from build123d import *

# Parameters (mm, degrees)
SKETCH1_W           = 8
SKETCH1_H           = 8
BOSS_EXTRUDE1_DEPTH = 2
SKETCH2_W           = 6
SKETCH2_H           = 6
BOSS_EXTRUDE2_DEPTH = 5
FILLET1_R           = 1
SKETCH3_W           = 4
SKETCH3_H           = 4
BOSS_EXTRUDE3_DEPTH = 2.2
FILLET2_R           = 0.5


with BuildPart() as part:
    # Sketch1 → Boss-Extrude1 (new body)
    with BuildSketch(Plane(origin=(0, 0, 0), x_dir=(1, 0, 0), z_dir=(0, 1, 0))):
        Rectangle(SKETCH1_W, SKETCH1_H)
    extrude(amount=BOSS_EXTRUDE1_DEPTH)

    # Sketch2 → Boss-Extrude2 (add)
    with BuildSketch(Plane(origin=(0, 2, 0), x_dir=(1, 0, 0), z_dir=(0, 1, 0))):
        Rectangle(SKETCH2_W, SKETCH2_H)
    extrude(amount=BOSS_EXTRUDE2_DEPTH)

    # Fillet1
    fillet1_edges = [part.edges().sort_by_distance(p)[0] for p in [
        (3, 4.5, 3),
        (3, 4.5, -3),
        (-3, 4.5, -3),
        (-3, 4.5, 3),
    ]]
    fillet(fillet1_edges, radius=FILLET1_R)

    # Sketch3 → Boss-Extrude3 (add)
    with BuildSketch(Plane(origin=(0, 0, 0), x_dir=(-1, 0, 0), z_dir=(0, -1, 0))):
        Rectangle(SKETCH3_W, SKETCH3_H)
    extrude(amount=BOSS_EXTRUDE3_DEPTH)

    # Fillet2
    fillet2_edges = [part.edges().sort_by_distance(p)[0] for p in [
        (3, 7, 0),
        (0, 7, 3),
        (0, 7, -3),
        (-3, 7, 0),
        (-2.707106781, 7, -2.707106781),
        (-2.707106781, 7, 2.707106781),
        (2.707106781, 7, -2.707106781),
        (2.707106781, 7, 2.707106781),
    ]]
    fillet(fillet2_edges, radius=FILLET2_R)


solid = part.part
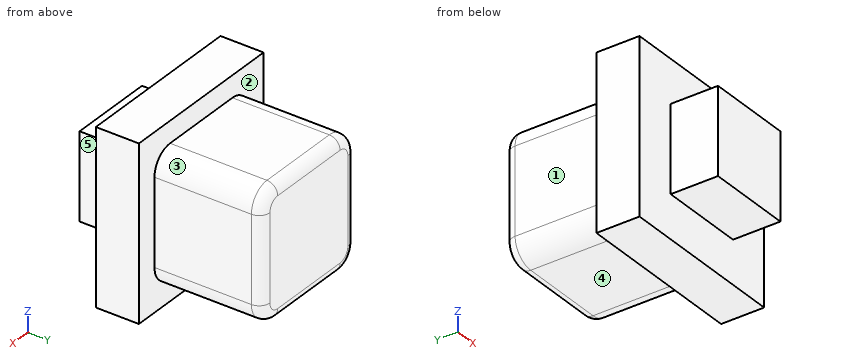
Read the model definition and answer for the solid it produces. Units are mm, in the model's axes. Face numbers are marked on the shaded views. A direction names the side the tool comes from. Give positions to 0.01 mm unless a question says otherwise; leave off trailing zeros. Loops run counter-clockwise (first coordinate to the right, second up) from the corner with the lowest first, then second, coordinate; pieces in that order, holes last. Notation, with made-up numbers: M 15.25,55.5 L 32.25,55.5 A17 ccw 32.25,60.5 Z; hole C -38,-36 d9. An arc over 180 degrees is marked long. Write each question's results on one line, items separated by ' | '.
1. Given pin 1 (1.2 mm diameter, centred on y = 3, z = 0, fed in from +X); pin 2 (3 mm diameter, centred on y = 4, z = 0, fed in from -X); pin 3 (2 mm diameter, centred on x = 0, y = 5, fed in from +Z), each flat-ended and moving along its own axis, determine where each tip first touches the part or whether it passes through.
Values:
pin 1: stops at x = 3 | pin 2: stops at x = -3 | pin 3: stops at z = 3
2. Straight lines are drawn through the part: line 1 (Y direction, x = 3.5, z = 1.5); line 2 (Y direction, x = 2.25, z = 2); line 3 (Z direction, x = 1.25, y = -1.75). For each, find the intervals that lie inside material, in ascending order. Write a range as [from, to].
Values:
line 1: y = [0, 2] | line 2: y = [0, 7] | line 3: z = [-2, 2]
3. Section C-C on y = 4.75 is taken. Give the vertices of the cut face in (x, z).
Values:
outline: M -3,-2 A1 ccw -2,-3 L 2,-3 A1 ccw 3,-2 L 3,2 A1 ccw 2,3 L -2,3 A1 ccw -3,2 Z
4. Section A-A on z = -1.75 is taken. Give the vertices of the cut face in (x, y), plus the area to 3 significant figures.
Values:
outline: M -4,0 L -2,0 L -2,-2.2 L 2,-2.2 L 2,0 L 4,0 L 4,2 L 3,2 L 3,6.5 A0.5 ccw 2.5,7 L -2.5,7 A0.5 ccw -3,6.5 L -3,2 L -4,2 Z | area: 54.7 mm^2
5. Section B-B on x = -0.5 is taken. Give the vertices of the cut face in (y, z).
Values:
outline: M -2.2,-2 L 0,-2 L 0,-4 L 2,-4 L 2,-3 L 6.5,-3 A0.5 ccw 7,-2.5 L 7,2.5 A0.5 ccw 6.5,3 L 2,3 L 2,4 L 0,4 L 0,2 L -2.2,2 Z
6. A tool of negligible diameter and unlimited length cuts with its end or side. For the marked faces 1, 2, 3, 4 and 5, from which of +Z, -Z, +X, -X, +Y, -Y can it reach the whole face along a straight path? Write none if from no direction.
Values:
face 1: +Z, -Z, -X, +Y | face 2: +Y | face 3: +Z, +X, +Y | face 4: -Z, +X, -X, +Y | face 5: +Z, -Z, +X, -Y
